The model under review builds one solid part; all positions refer to its coordinate system, in mm. A direction names the side the tool comes from. Round coordinates to 2 decimals unless told otherwise and drop trailing zeros. Loops run counter-clockwise (first coordinate to the right, second up) from the corner with the lowest first, then second, coordinate; pieces in that order, holes last. Notation, with made-up numbers: M -17.75,29.25 L -8.75,29.25 A12 cw -8.75,34.25 Z; hole C 75.5,-23.5 d2. An arc over 180 degrees is marked long. Return JSON: item names as keys, results as strings. Group by question number.
Q1. To check wall thickness, follow line 1 along X through (y, z) = (2.35, -11.65); line 2 along Y through (x, z) = (54.65, -11.65); line 3 along Z through (x, y) = (54, -18). State the ranges of each line that lie inside material, in increasing order.
Q2. Consider section C-C (z = -4.65). State the section outline as (x, y) points.
Q3. For faces 1 (the face through (27, 0, -17)), 2 (the face through (54.46, -26.94, -3.28)), list the 3-axis set-ups (+Z, -Z, +X, -X, +Y, -Y) from which the entire face can be reached by the end or side of a thin tool; tool diameter is ignored.
Q4. Draft analysis for pull direction X (two halves, no side actions). For faces 3 (the face through (0.542, -26.283, -10.726)), 4 (the face through (55, -9, -12)), 5 (the face through (0, -13, -11)), 6 (the face through (33.49, 2.33, -6.01)), state which applies: pulls with the +X half, pulls with the -X half, needs draft (parallel to the pull), parting line crosses it, or undercut.
Q5. Clearance check with a flat-ended pin moving along its axis: pin 1 Ø6 at (x, z) = (8, -18) entering from -Y. State where the tip first meets the part, or that it passes through.
Q6. Consider section A-A (x = 42.41). State the section outline as (y, z) points.
Q7. Consider section D-D (y = -25.9). State the section outline as (x, z) points, and give its area (3 significant figures).
Q8. Consider section B-B (y = -10). State the section outline as (x, z) points.
from build123d import *

# Parameters (mm, degrees)
SKETCH1_W                = 55
SKETCH1_H                = 23.3
MOUNTPLATE_DEPTH         = 4.6
SKETCH3_R                = 4.5
AXLEHOLE_MOUNT_DEPTH     = 4.6
SKETCH2_R                = 1
MOUNTHOLES_DEPTH         = 4.6
SKETCH4_W                = 1.1
SKETCH4_H                = 23.3
SERVOLEGS_DEPTH          = 30.4
CENTERHOLES_REACH        = 69.023
SKETCH5_R                = 4.5
ROTATOR_MOUNTHOLES_REACH = 69.023
SKETCH6_R                = 1
FILLET1_R                = 11.5
FILLET2_R                = 11.5
FILLET3_R                = 11.5
FILLET4_R                = 11.5


with BuildPart() as part:
    # Sketch1 → MountPlate (new body)
    with BuildSketch(Plane(origin=(0, 0, 0), x_dir=(1, 0, 0), z_dir=(0, 1, 0))):
        with Locations((27.5, 11.65)):
            Rectangle(SKETCH1_W, SKETCH1_H)
    extrude(amount=MOUNTPLATE_DEPTH)

    # Sketch3 → AxleHole-Mount (cut)
    with BuildSketch(Plane(origin=(0, 4.6, 0), x_dir=(1, 0, 0), z_dir=(0, 1, 0))):
        with Locations(Location((27.5, 11.65, 0), (0, 0, 270))):
            Circle(SKETCH3_R)
    extrude(amount=-AXLEHOLE_MOUNT_DEPTH, mode=Mode.SUBTRACT)

    # Sketch2 → MountHoles (cut)
    with BuildSketch(Plane(origin=(0, 4.6, 0), x_dir=(1, 0, 0), z_dir=(0, 1, 0))):
        with Locations(Location((22.35, 16.75, 0), (0, 0, 270))):
            Circle(SKETCH2_R)
        with Locations(Location((12.59, 11.65, 0), (0, 0, 270))):
            Circle(SKETCH2_R)
        with Locations(Location((32.65, 16.75, 0), (0, 0, 270))):
            Circle(SKETCH2_R)
        with Locations(Location((22.35, 6.55, 0), (0, 0, 270))):
            Circle(SKETCH2_R)
        with Locations(Location((42.41, 11.65, 0), (0, 0, 270))):
            Circle(SKETCH2_R)
        with Locations(Location((32.65, 6.55, 0), (0, 0, 270))):
            Circle(SKETCH2_R)
    extrude(amount=-MOUNTHOLES_DEPTH, mode=Mode.SUBTRACT)

    # Sketch4 → ServoLegs (add)
    with BuildSketch(Plane.XZ):
        with Locations((54.45, -11.65)):
            Rectangle(SKETCH4_W, SKETCH4_H)
        with Locations((0.55, -11.65)):
            Rectangle(SKETCH4_W, SKETCH4_H)
    extrude(amount=SERVOLEGS_DEPTH)

    # CenterHoles: up to this face of the body (flat: up to its plane)
    centerholes_end = Plane(part.part.faces().sort_by_distance((55, -12.9, -11.65))[0])
    # Sketch5 → CenterHoles (cut, up to the picked face)
    with BuildSketch(Plane.ZY, mode=Mode.PRIVATE) as centerholes_sk1:
        with Locations((-11.65, -18.9)):
            Circle(SKETCH5_R)
    centerholes_tool1 = split(extrude(centerholes_sk1.sketch, amount=-CENTERHOLES_REACH, mode=Mode.PRIVATE), bisect_by=centerholes_end, keep=Keep.BOTH, mode=Mode.PRIVATE)
    add(centerholes_tool1.solids().sort_by(Axis((0, -18.9, -11.65), (1, 0, 0)))[0], mode=Mode.SUBTRACT)

    # Rotator-MountHoles: up to this face of the body (flat: up to its plane)
    rotator_mountholes_end = Plane(part.part.faces().sort_by_distance((55, -12.392336394, -11.65))[0])
    # Sketch6 → Rotator-MountHoles (cut, up to the picked face)
    with BuildSketch(Plane.ZY, mode=Mode.PRIVATE) as rotator_mountholes_sk1:
        with Locations((-11.65, -25.9)):
            Circle(SKETCH6_R)
    rotator_mountholes_tool1 = split(extrude(rotator_mountholes_sk1.sketch, amount=-ROTATOR_MOUNTHOLES_REACH, mode=Mode.PRIVATE), bisect_by=rotator_mountholes_end, keep=Keep.BOTH, mode=Mode.PRIVATE)
    # Sketch6 → Rotator-MountHoles (cut, up to the picked face)
    with BuildSketch(Plane.ZY, mode=Mode.PRIVATE) as rotator_mountholes_sk2:
        with Locations((-18.65, -18.9)):
            Circle(SKETCH6_R)
    rotator_mountholes_tool2 = split(extrude(rotator_mountholes_sk2.sketch, amount=-ROTATOR_MOUNTHOLES_REACH, mode=Mode.PRIVATE), bisect_by=rotator_mountholes_end, keep=Keep.BOTH, mode=Mode.PRIVATE)
    # Sketch6 → Rotator-MountHoles (cut, up to the picked face)
    with BuildSketch(Plane.ZY, mode=Mode.PRIVATE) as rotator_mountholes_sk3:
        with Locations((-11.65, -11.9)):
            Circle(SKETCH6_R)
    rotator_mountholes_tool3 = split(extrude(rotator_mountholes_sk3.sketch, amount=-ROTATOR_MOUNTHOLES_REACH, mode=Mode.PRIVATE), bisect_by=rotator_mountholes_end, keep=Keep.BOTH, mode=Mode.PRIVATE)
    # Sketch6 → Rotator-MountHoles (cut, up to the picked face)
    with BuildSketch(Plane.ZY, mode=Mode.PRIVATE) as rotator_mountholes_sk4:
        with Locations((-4.65, -18.9)):
            Circle(SKETCH6_R)
    rotator_mountholes_tool4 = split(extrude(rotator_mountholes_sk4.sketch, amount=-ROTATOR_MOUNTHOLES_REACH, mode=Mode.PRIVATE), bisect_by=rotator_mountholes_end, keep=Keep.BOTH, mode=Mode.PRIVATE)
    add(rotator_mountholes_tool1.solids().sort_by(Axis((0, -25.9, -11.65), (1, 0, 0)))[0], mode=Mode.SUBTRACT)
    add(rotator_mountholes_tool2.solids().sort_by(Axis((0, -18.9, -18.65), (1, 0, 0)))[0], mode=Mode.SUBTRACT)
    add(rotator_mountholes_tool3.solids().sort_by(Axis((0, -11.9, -11.65), (1, 0, 0)))[0], mode=Mode.SUBTRACT)
    add(rotator_mountholes_tool4.solids().sort_by(Axis((0, -18.9, -4.65), (1, 0, 0)))[0], mode=Mode.SUBTRACT)

    # Fillet1
    fillet1_edges = [part.edges().sort_by_distance(p)[0] for p in [
        (0.55, -30.4, -23.3),
    ]]
    fillet(fillet1_edges, radius=FILLET1_R)

    # Fillet2
    fillet2_edges = [part.edges().sort_by_distance(p)[0] for p in [
        (0.55, -30.4, 0),
    ]]
    fillet(fillet2_edges, radius=FILLET2_R)

    # Fillet3
    fillet3_edges = [part.edges().sort_by_distance(p)[0] for p in [
        (54.45, -30.4, 0),
    ]]
    fillet(fillet3_edges, radius=FILLET3_R)

    # Fillet4
    fillet4_edges = [part.edges().sort_by_distance(p)[0] for p in [
        (54.45, -30.4, -23.3),
    ]]
    fillet(fillet4_edges, radius=FILLET4_R)


solid = part.part
Values:
{
 "1": {"line 1": "x = 0 to 11.59, 13.59 to 23, 32 to 41.41, 43.41 to 55", "line 2": "y = -30.4 to -26.9, -24.9 to -23.4, -14.4 to -12.9, -10.9 to 4.6", "line 3": "z = -23.3 to -19.09, -18.21 to -16.06, -7.24 to -5.09, -4.21 to 0"},
 "2": {"outline": "M 0,-28.14 L 1.1,-28.14 L 1.1,-19.9 L 0,-19.9 Z; M 0,-17.9 L 1.1,-17.9 L 1.1,0 L 53.9,0 L 53.9,-17.9 L 55,-17.9 L 55,4.6 L 0,4.6 Z; M 53.9,-28.14 L 55,-28.14 L 55,-19.9 L 53.9,-19.9 Z"},
 "3": {"face 1": "+Z, -Z, -Y", "face 2": "+Z, +X, -X, -Y"},
 "4": {"face 3": "needs draft", "face 4": "pulls with the +X half", "face 5": "pulls with the -X half", "face 6": "undercut"},
 "5": {"pin 1": "stops at y = 0"},
 "6": {"outline": "M 0,-23.3 L 4.6,-23.3 L 4.6,-12.65 L 0,-12.65 Z; M 0,-10.65 L 4.6,-10.65 L 4.6,0 L 0,0 Z"},
 "7": {"outline": "M 0,-20.92 L 1.1,-20.92 L 1.1,-12.65 L 0,-12.65 Z; M 0,-10.65 L 1.1,-10.65 L 1.1,-2.38 L 0,-2.38 Z; M 53.9,-20.92 L 55,-20.92 L 55,-12.65 L 53.9,-12.65 Z; M 53.9,-10.65 L 55,-10.65 L 55,-2.38 L 53.9,-2.38 Z", "area": "36.4 mm2"},
 "8": {"outline": "M 0,-23.3 L 1.1,-23.3 L 1.1,0 L 0,0 Z; M 53.9,-23.3 L 55,-23.3 L 55,0 L 53.9,0 Z"}
}
